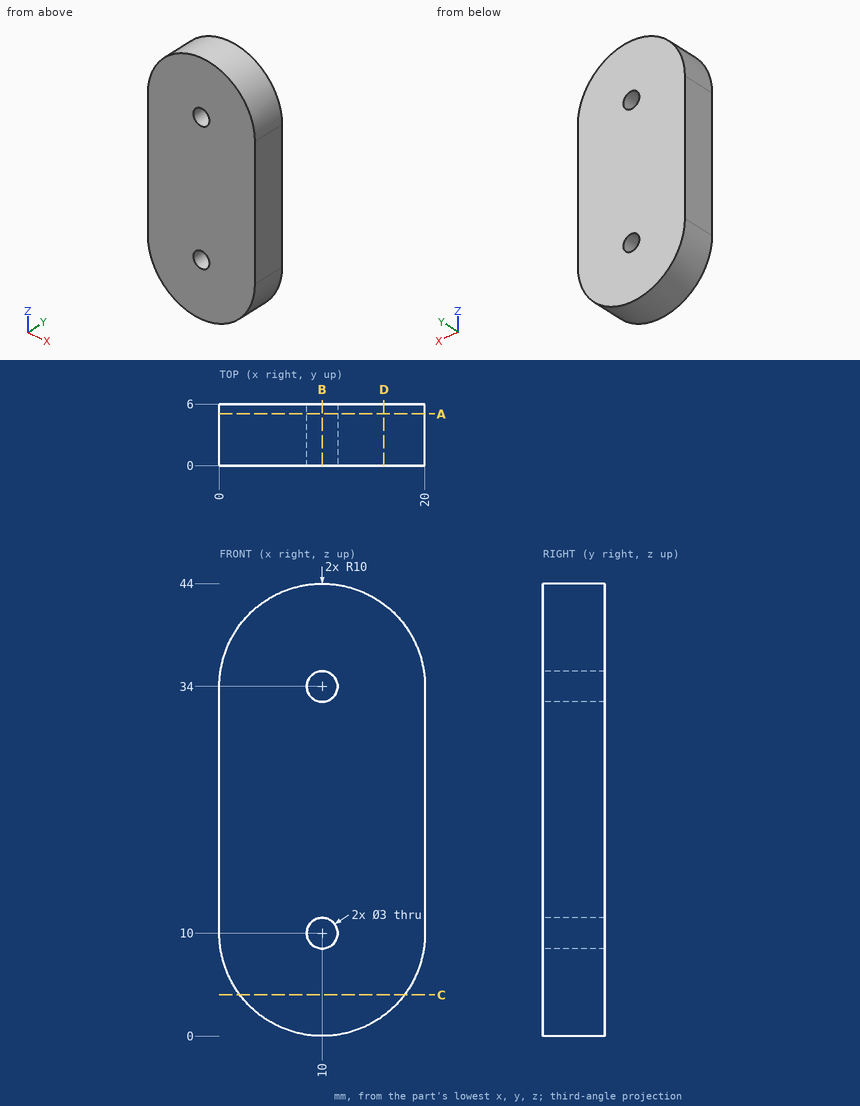
Source: three-view drawing plus pictorial views. Frame: mm from the lowest corner of the part. Give positions to 0.01 mm unless a question says otherwise; leave off trailing zeros. Write each loop counter-clockwise with the first axis right and the second up, starting at its lowest first coordinate (ties: lowest second). Pieces come first, ordered by that corner, then holes.
(1) Ray query, line 1 (Z direction, x = 10, y = 1.45); line 2 (X direction, y = 2.5, z = 10); line 3 (Z direction, x = 9, y = 1.1). Return the intervals inside material, ascending.
(2) Cut plane D-D, the plane x = 16. Return loops of the section in (y, z).
(3) First-contact query: P1, Ø8, axis at x = 4.5, z = 27, coming from the -Y side; P2, Ø1.5, axis at x = 7.5, y = 4, coming from the +Z side; P3, Ø2.5, axis at x = 10, z = 10, coming from the -Y side. Flat tips, straight axial feed; report the tip coordinate or a pass-through.
(4) Cut plane C-C, the plane z = 4. Return loops of the section in (x, y).
(5) Cut plane B-B, the plane x = 10. Return loops of the section in (y, z), then the cut area to 3 significant figures.
(6) Cut plane A-A, the plane y = 5.05. Return loops of the section in (x, z), then the cut area to 3 significant figures.
Values follow:
1. line 1: z = 0 to 8.5, 11.5 to 32.5, 35.5 to 44
1. line 2: x = 0 to 8.5, 11.5 to 20
1. line 3: z = 0.05 to 8.88, 11.12 to 32.88, 35.12 to 43.95
2. outline: (0, 2) - (6, 2) - (6, 42) - (0, 42) - close
3. P1: stops at y = 0
3. P2: stops at z = 43.85
3. P3: passes through
4. outline: (2, 0) - (18, 0) - (18, 6) - (2, 6) - close
5. outline: (0, 0) - (6, 0) - (6, 8.5) - (0, 8.5) - close; (0, 11.5) - (6, 11.5) - (6, 32.5) - (0, 32.5) - close; (0, 35.5) - (6, 35.5) - (6, 44) - (0, 44) - close
5. area: 228 mm2
6. outline: (0, 10) arc R10 ccw to (20, 10) - (20, 34) arc R10 ccw to (0, 34) - close; hole circle Ø3 at (10, 10); hole circle Ø3 at (10, 34)
6. area: 780 mm2
